The figure shows three views and two pictorial views of one solid part (mm, origin at its lowest corner). Answer the questions. A direction names the side the tool comes from. Coordinates: 2 decimals unless noted, no trailing zeros. Write each loop counter-clockwise with the first axis right and the second up, starting at its lowest first coordinate (ties: lowest second). Pieces come first, ordered by that corner, then holes. Notation, with made-up numbers: M 28,88 L 64,88 A10 ccw 64,93 Z; hole C -29,8 d1. An arc over 180 degrees is marked long. Use CSV: the item, a comma, the result in double quotes.
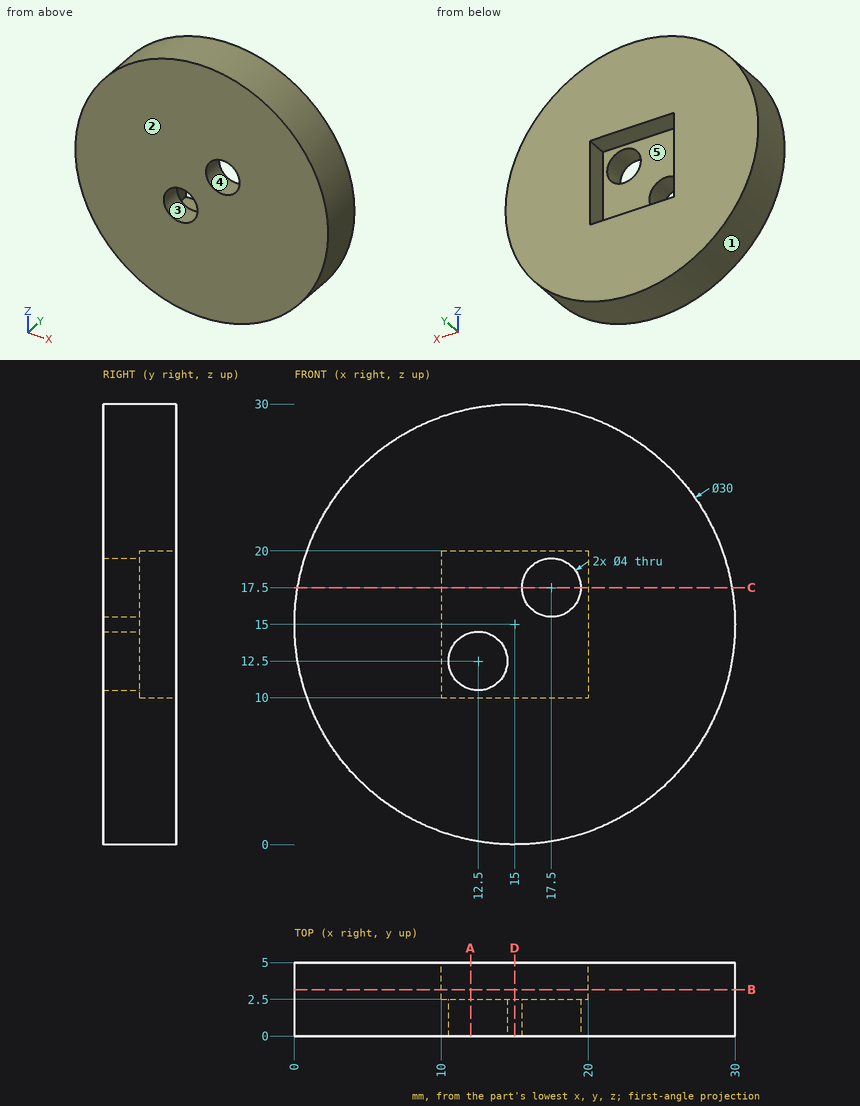
Item 1: The part is cut by section A-A (x = 12). Write down the section's boundary in (y, z).
Answer:
outline,"M 0,0.3 L 5,0.3 L 5,10 L 2.5,10 L 2.5,10.56 L 0,10.56 Z; M 0,14.44 L 2.5,14.44 L 2.5,20 L 5,20 L 5,29.7 L 0,29.7 Z"
Item 2: The part is cut by section D-D (x = 15). Write down the section's boundary in (y, z).
Answer:
outline,"M 0,0 L 5,0 L 5,10 L 2.5,10 L 2.5,20 L 5,20 L 5,30 L 0,30 Z"
Item 3: The part is cut by section B-B (y = 3.15). Write down the section's boundary in (x, z), then the cut area to 3 significant figures.
Answer:
outline,"C 15,15 d30; hole M 10,10 L 20,10 L 20,20 L 10,20 Z"
area,"607 mm2"
Item 4: A tool of negligible diameter and unlimited length cuts with its end or side. For the marked faces 4 and 5, from which of +Z, -Z, +X, -X, +Y, -Y can it reach the whole face along a straight path? Write none if from no direction.
Answer:
face 4,"+Y, -Y"
face 5,"+Y"
Item 5: The part is cut by section C-C (z = 17.5). Write down the section's boundary in (x, y), then the cut area to 3 significant figures.
Answer:
outline,"M 0.21,0 L 15.5,0 L 15.5,2.5 L 10,2.5 L 10,5 L 0.21,5 Z; M 19.5,0 L 29.79,0 L 29.79,5 L 20,5 L 20,2.5 L 19.5,2.5 Z"
area,"113 mm2"
Item 6: For a pull along Z with two mould halves and no side action, classify the marked faces 1, 2 and 3 as released by +Z, released by -Z, zero draft, split by the parting line, or undercut.
Answer:
face 1,"split by the parting line"
face 2,"zero draft"
face 3,"undercut"
Item 7: Given pin 1 (0.8 mm diameter, centred on x = 16, y = 4.5, fed in from -Z); pin 2 (2 mm diameter, centred on x = 13.5, y = 4, fed in from +Z); pin 3 (3 mm diameter, centred on x = 14.5, z = 13, fed in from +Y); pin 4 (4.5 mm diameter, centred on x = 17.5, z = 17.5, fed in from -Y), each flat-ended and moving along its own axis, determine where each tip first touches the part or whether it passes through.
Answer:
pin 1,"stops at z = 0.01"
pin 2,"stops at z = 29.99"
pin 3,"stops at y = 2.5"
pin 4,"stops at y = 0"
Item 8: Consider probe 1 along Z at (x, y) = (18.25, 4.85); probe 2 along X at (y, z) = (1.3, 17.5); probe 3 along Z at (x, y) = (16.75, 3.4). Determine where each line is inside the solid, lowest interval first.
Answer:
probe 1,"z = 0.36 to 10, 20 to 29.64"
probe 2,"x = 0.21 to 15.5, 19.5 to 29.79"
probe 3,"z = 0.1 to 10, 20 to 29.9"
